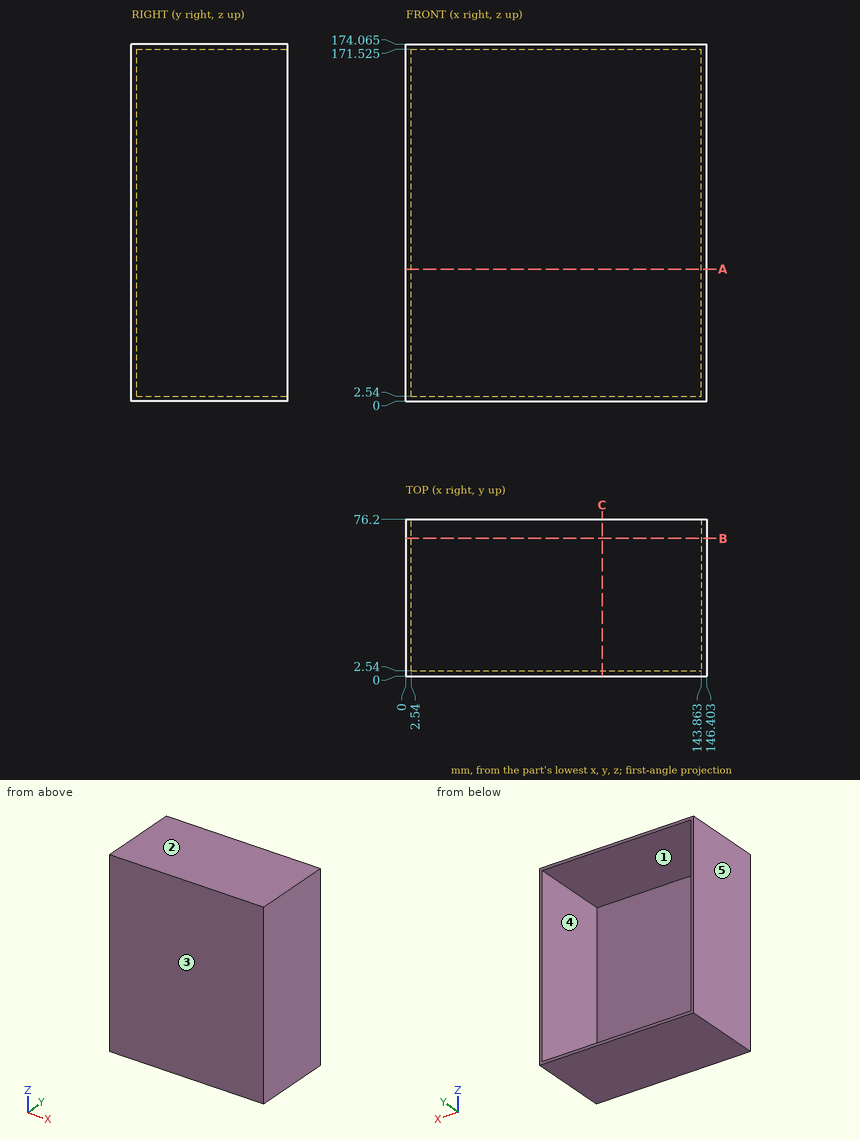
Geometry check sheet. Reference: drawing and pictorial views, mm from the part's lowest x, y, z. A direction names the side the tool comes from. Give positions to 0.01 mm unless a question says otherwise; leave off trailing zeros. Loops run counter-clockwise (first coordinate to the right, second up) from the corner with the lowest first, then second, coordinate; pieces in that order, holes last. Notation, with made-up numbers: M 86,15.5 L 97,15.5 A24 ccw 97,37.5 Z; hole C 32,-32.75 d1. An arc over 180 degrees is marked long. Use a Markdown table: item, result. Add a question column.
Q1. Mould release check, pull along Z, two halves, no side actions. Record for the marked faces 1, 2 and 3: pulls with the +Z half, pulls with the -Z half, needs draft (parallel to the pull), parting line crosses it, or undercut.
Q2. Scan lines: line 1 along X through (y, z) = (30, 113); line 2 along Z through (x, y) = (20.5, 40.5) (1 decimal); line 3 along Y through (x, z) = (103, 89). Record each from-to range of solid material in increasing order. Write a range as [from, to].
Q3. Sectioned sample at C-C, the plane x = 95.5. Record the cut outline in (y, z) (1 decimal).
Q4. Go/stop test with a flat-tipped pin: pin 1 (8 mm diameter, centred on x = 73.5, z = 98, fed in from +Y). Record where the tip stops, or that it passes through.
Q5. Sectioned sample at B-B, the plane y = 67. Record the cut outline in (x, z) (1 decimal).
Q6. Tool access check on the marked faces 4 and 5. Record the directions out of +Z, -Z, +X, -X, +Y, -Y that give a thin tool (end or side, any length) a straight path to the whole face; none if there is none.
Q7. Sectioned sample at A-A, the plane z = 64.5. Record the cut outline in (x, y).
Verdict:
| question | item | result |
|---|---|---|
| 1 | face 1 | undercut |
| 1 | face 2 | pulls with the +Z half |
| 1 | face 3 | needs draft |
| 2 | line 1 | [0, 2.54], [143.86, 146.4] |
| 2 | line 2 | [0, 2.5], [171.5, 174.1] |
| 2 | line 3 | [0, 2.54] |
| 3 | outline | M 0,0 L 76.2,0 L 76.2,2.5 L 2.5,2.5 L 2.5,171.5 L 76.2,171.5 L 76.2,174.1 L 0,174.1 Z |
| 4 | pin 1 | y = 2.54 |
| 5 | outline | M 0,0 L 146.4,0 L 146.4,174.1 L 0,174.1 Z; hole M 2.5,2.5 L 143.9,2.5 L 143.9,171.5 L 2.5,171.5 Z |
| 6 | face 4 | +Y |
| 6 | face 5 | +Z, -Z, -X, +Y, -Y |
| 7 | outline | M 0,0 L 146.4,0 L 146.4,76.2 L 143.86,76.2 L 143.86,2.54 L 2.54,2.54 L 2.54,76.2 L 0,76.2 Z |
